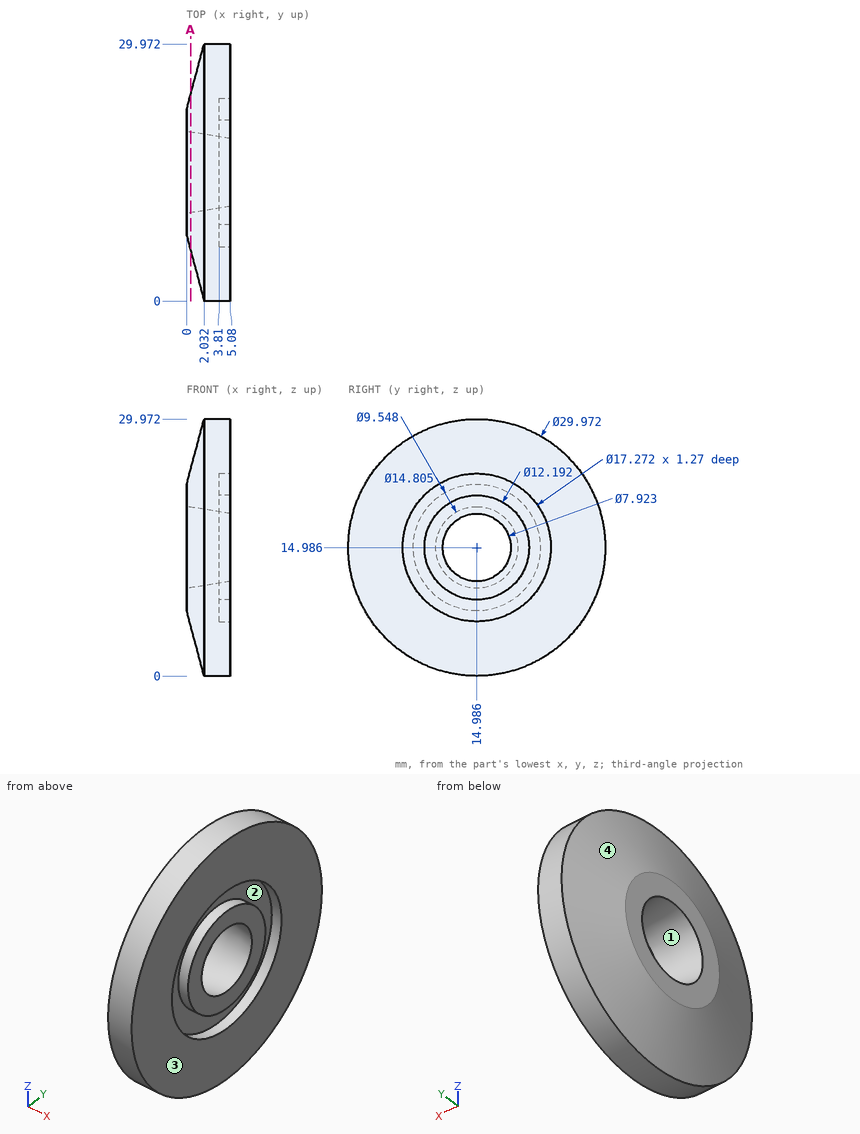
Geometry check sheet. Reference: drawing and pictorial views, mm from the part's lowest x, y, z. Round coordinates to 2 decimals unless told otherwise and drop trailing zeros. Write each loop counter-clockwise with the first axis right and the second up, starting at its lowest first coordinate (ties: lowest second). Pieces come first, ordered by that corner, then holes. Notation, with made-up numbers: (-19, -20.5) -> (29, -20.5) arc R18 cw to (29, -7.5) -> close; hole circle Ø6 at (32.25, 75.25). An arc over 180 degrees is marked (long way). One line per question, with ' | ' between items. Start each with the question number.
1. Sectioned sample at A-A, the plane x = 0.45. Record the cut outline in (y, z).
2. Scan lines: line 1 along Z through (x, y) = (4.1, 14.5); line 2 along X through (y, z) = (22.25, 16.5) (1 decimal); line 3 along Y through (x, z) = (3.3, 14.5). Record each from-to range of solid material in increasing order. Write a range as from..to.
3. Release check for a two-part mould opening along Z. For the marked faces 1, 2, 3 and 4 record: +Z half, -Z half, draft (parallel to the pull), parting line (faces both ways), or undercut.
4. Depth check by flat-ended pin: pin 1 (3 mm diameter, centred on x = 3.5, z = 19, fed in from +Y); pin 2 (2 mm diameter, centred on x = 2.5, z = 23.5, fed in from -Y); pin 3 (5 mm diameter, centred on y = 16, z = 14.5, fed in from +X). Enter the tip coordinate at first touch or a pass-through.
Taken from the geometry:
1) outline: circle Ø18.16 at (14.99, 14.99); hole circle Ø9.4 at (14.99, 14.99)
2) line 1: z = 0.01..6.36, 8.91..10.9, 19.08..21.06, 23.61..29.96 | line 2: x = 0..3.8 | line 3: y = 0.01..10.77, 19.2..29.96
3) face 1: undercut | face 2: undercut | face 3: draft | face 4: parting line
4) pin 1: stops at y = 29.76 | pin 2: stops at y = 2.02 | pin 3: passes through
